Autodesk Inventor part; units mm, degrees
ref_plane "YZ Plane" through (0, 0, 0) normal (1, 0, 0) x (0, 1, 0)
ref_plane "XZ Plane" through (0, 0, 0) normal (0, 1, 0) x (-1, 0, 0)
ref_plane "XY Plane" through (0, 0, 0) normal (0, 0, 1) x (1, 0, 0)
sketch "Sketch1" plane through (0, 0, 0) normal (0, 0, 1) x (1, 0, 0)
  line L0 (2.54, -4.344) -> (-2.54, -4.344)
  line L1 (-2.54, -4.344) -> (-2.54, 4.344)
  line L2 (-2.54, 4.344) -> (2.54, 4.344)
  line L3 (2.54, 4.344) -> (2.54, -4.344)
  line L4 (2.54, -4.344) -> (-2.54, 4.344) construction
  line L5 (-2.54, -4.344) -> (2.54, 4.344) construction
  line L6 (4.445, 6.884) -> (-4.445, 6.884)
  line L7 (-4.445, 6.884) -> (-4.445, 1.804)
  line L8 (-4.445, 1.804) -> (4.445, 1.804)
  line L9 (4.445, 1.804) -> (4.445, 6.884)
  line L10 (4.445, 6.884) -> (-4.445, 1.804) construction
  line L11 (-4.445, 6.884) -> (4.445, 1.804) construction
  line L12 (3.8177, 1.5502) -> (-3.8177, 7.1379) construction
  line L13 (-4.445, -1.73) -> (4.445, 10.418) construction
  line L14 (6.985, 0) -> (-6.985, 0)
  line L15 (-6.985, 0) -> (-6.985, 25.4)
  line L16 (-6.985, 25.4) -> (6.985, 25.4)
  line L17 (6.985, 25.4) -> (6.985, 0)
  line L18 (6.985, 0) -> (-6.985, 25.4) construction
  line L19 (-6.985, 0) -> (6.985, 25.4) construction
  line L20 (0, 25.4) -> (0, 0) construction
  line L21 (-1.5875, 25.4) -> (1.5875, 25.4)
  line L22 (1.5875, 25.4) -> (1.5875, 13.234)
  line L23 (1.5875, 13.234) -> (-1.5875, 13.234)
  line L24 (-1.5875, 13.234) -> (-1.5875, 25.4)
  point P0 (0, 4.344)
  point P1 (0, 12.7)
  point P2 (2.54, 1.804)
  point P3 (2.54, 0)
  point P4 (-2.54, 0)
  point P5 (-2.54, 1.804)
  dimension "d0" = 5.08
  dimension "d1" = 8.89
  dimension "d2" = 5.08
  dimension "d3" = 8.89
  dimension "d4" = 8.89
  dimension "d5" = 13.97
  dimension "d6" = 25.4
  dimension "d7" = 0
  dimension "d8" = 3.175
  dimension "d9" = 1.5875
  dimension "d27" = 6.35
extrude "Extrusion1" add sketch "Sketch1" along normal blind 44.45 contours L3 L8 L9 L6 L7 L1 L14 L15 L16 L24 L23 L22 L17
sketch "Sketch2" plane through (0, 0, 0) normal (0, 0, -1) x (-1, 0, 0)
  line L0 (4.445, 6.884) -> (-4.445, 6.884)
  line L1 (4.445, 1.804) -> (4.445, 6.884)
  line L2 (2.54, 1.804) -> (4.445, 1.804)
  line L3 (2.54, 0) -> (2.54, 1.804)
  line L4 (6.985, 0) -> (2.54, 0)
  line L5 (6.985, 25.4) -> (6.985, 0)
  line L6 (1.5875, 25.4) -> (6.985, 25.4)
  line L7 (1.5875, 13.234) -> (1.5875, 25.4)
  line L8 (-1.5875, 13.234) -> (1.5875, 13.234)
  line L9 (-1.5875, 25.4) -> (-1.5875, 13.234)
  line L10 (-6.985, 25.4) -> (-1.5875, 25.4)
  line L11 (-6.985, 0) -> (-6.985, 25.4)
  line L12 (-2.54, 0) -> (-6.985, 0)
  line L13 (-2.54, 1.804) -> (-2.54, 0)
  line L14 (-4.445, 1.804) -> (-2.54, 1.804)
  line L15 (-4.445, 6.884) -> (-4.445, 1.804)
  line L16 (-1.5875, 25.4) -> (1.5875, 25.4)
  line L17 (1.5875, 25.4) -> (1.5875, 13.234)
  line L18 (1.5875, 13.234) -> (-1.5875, 13.234)
  line L19 (-1.5875, 13.234) -> (-1.5875, 25.4)
  point P0 (0, 0)
  point P1 (1.5875, 25.4)
extrude "Extrusion2" add sketch "Sketch2" against normal blind 6.35 contours L7 L8 L9 L16
sketch "Sketch3" plane through (6.985, 0, 0) normal (1, 0, 0) x (0, 0, -1)
  line L0 (0, 0) -> (0, 25.4)
  line L1 (0, 25.4) -> (-44.45, 25.4)
  line L2 (-44.45, 0) -> (-44.45, 25.4)
  line L3 (0, 0) -> (-44.45, 0)
  line L4 (-6.35, 25.4) -> (-6.35, 13.234)
  circle A0 centre (-3.175, 15.24) radius 3.175
  point P0 (0, 0)
  point P1 (0, 12.7)
  dimension "d14" = 6.35
  dimension "d15" = 3.175
  dimension "d16" = 10.16
extrude "Extrusion3" cut sketch "Sketch3" against normal through all contours A0
sketch "Sketch4" plane through (0, 0, 0) normal (0, 0, -1) x (-1, 0, 0)
  line L0 (4.445, 6.884) -> (-4.445, 6.884)
  line L1 (4.445, 1.804) -> (4.445, 6.884)
  line L2 (2.54, 1.804) -> (4.445, 1.804)
  line L3 (2.54, 0) -> (2.54, 1.804)
  line L4 (6.985, 0) -> (2.54, 0)
  line L5 (6.985, 25.4) -> (6.985, 15.24)
  line L6 (-6.985, 25.4) -> (6.985, 25.4)
  line L7 (-6.985, 0) -> (-6.985, 15.24)
  line L8 (-2.54, 0) -> (-6.985, 0)
  line L9 (-2.54, 1.804) -> (-2.54, 0)
  line L10 (-4.445, 1.804) -> (-2.54, 1.804)
  line L11 (-4.445, 6.884) -> (-4.445, 1.804)
  line L12 (-6.985, 0) -> (-6.985, 25.4)
  line L13 (-6.985, 12.7) -> (6.985, 12.7)
  line L14 (6.985, 25.4) -> (6.985, 0)
  line L15 (-6.985, 15.24) -> (6.985, 15.24)
  line L16 (-6.985, 15.24) -> (-6.985, 25.4)
  line L17 (6.985, 15.24) -> (6.985, 0)
  point P0 (0, 0)
  point P1 (-6.985, 12.7)
  point P2 (6.985, 12.7)
  dimension "d19" = 12.7
extrude "Extrusion4" add sketch "Sketch4" along normal blind 6.35
sketch "Sketch5" plane through (-6.985, 25.4, 44.45) normal (0, 1, 0) x (1, 0, 0)
  line L0 (0, 50.8) -> (0, 0)
  line L1 (13.97, 50.8) -> (13.97, 0)
  line L2 (0, 50.8) -> (13.97, 50.8)
  line L3 (13.97, 50.8) -> (13.97, 40.64)
  line L4 (13.97, 40.64) -> (0, 40.64)
  line L5 (0, 40.64) -> (0, 50.8)
  line L6 (0, 48.26) -> (13.97, 48.26)
  line L7 (13.97, 48.26) -> (13.97, 43.18)
  line L8 (13.97, 43.18) -> (0, 43.18)
  line L9 (0, 43.18) -> (0, 48.26)
  line L10 (0, 48.26) -> (13.97, 43.18) construction
  line L11 (13.97, 48.26) -> (0, 43.18) construction
  point P0 (6.985, 44.45)
  point P1 (6.985, 45.72)
  point P2 (0, 43.18)
  dimension "d22" = 10.16
  dimension "d23" = 5.08
  dimension "d24" = 5.08
  dimension "d29" = 0
extrude "Extrusion5" cut sketch "Sketch5" against normal blind 8.89 contours L6 L1 L8 L0
fillet "Fillet1" [suppressed]
properties part number "Drone_Launcher_Carriage"
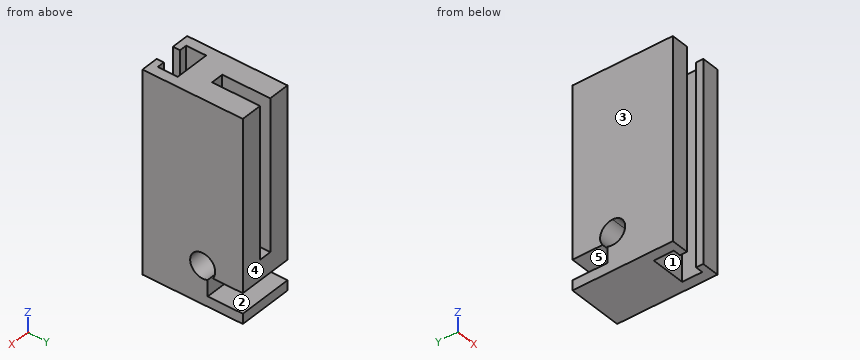
The listing builds one solid part. Answer for the finished solid, in the listing's coordinates (mm). Face numbers are marked on the shaded views. A direction names the side the tool comes from. Give positions to 0.01 mm unless a question says otherwise; leave off trailing zeros. Write each loop counter-clockwise with the first axis right and the second up, starting at its lowest first coordinate (ties: lowest second). Pieces come first, ordered by that corner, then holes. Notation, with made-up numbers: (73, 15.25) - (93, 15.25) arc R24 ccw to (93, 45.25) - close; hole circle Ø8 at (22.25, -37.75). An arc over 180 degrees is marked (long way). Use a Markdown table: item, result.
1. Find the intervals of material crossed by probe 1 along Z at (x, y) = (5, 20.75); probe 2 along Y at (x, z) = (-3.75, 39.5); probe 3 along X at (y, z) = (2.5, 31.5) (3 decimals), in increasing order. Write a range as from..to.
Values follow:
| item | result |
|---|---|
| probe 1 | z = -6.35..-3.81, 1.27..44.45 |
| probe 2 | y = 0..1.8, 6.88..25.4 |
| probe 3 | x = -6.985..-4.445, 4.445..6.985 |
2. Section D-D on z = 3.5 is taken. Write down the section's boundary in (x, y) (3 decimals), plus the area to 3 significant figures.
Values follow:
| item | result |
|---|---|
| outline | (-6.985, 0) - (-2.54, 0) - (-2.54, 1.804) - (-4.445, 1.804) - (-4.445, 6.884) - (4.445, 6.884) - (4.445, 1.804) - (2.54, 1.804) - (2.54, 0) - (6.985, 0) - (6.985, 12.082) - (-6.985, 12.082) - close; (-6.985, 18.398) - (6.985, 18.398) - (6.985, 25.4) - (-6.985, 25.4) - close |
| area | 212 mm² |
3. For a pull along X with two mould halves and no side action, classify the marked faces 1, 2 and 3 as released by +X, released by -X, zero draft, split by the parting line, or undercut.
Values follow:
| item | result |
|---|---|
| face 1 | undercut |
| face 2 | zero draft |
| face 3 | released by -X |
4. Section A-A on y = 2.75 is taken. Write down the section's boundary in (x, z) (3 decimals), plus the area to 3 significant figures.
Values follow:
| item | result |
|---|---|
| outline | (-6.985, -6.35) - (-4.445, -6.35) - (-4.445, 44.45) - (-6.985, 44.45) - close; (4.445, -6.35) - (6.985, -6.35) - (6.985, 44.45) - (4.445, 44.45) - close |
| area | 258 mm² |
5. A tool of negligible diameter and unlimited length cuts with its end or side. For the marked faces 4 and 5, from which of +Z, -Z, +X, -X, +Y, -Y can it reach the whole face along a straight path? Write none if from no direction.
Values follow:
| item | result |
|---|---|
| face 4 | +Z, -Z, +X, -X, +Y |
| face 5 | +X, -X, +Y |
6. Each of these flat-tipped pins is pushed along its axis until it touches: P1, Ø4, axis at x = -4.5, z = 19.5, coming from the -Y side; P2, Ø1, axis at x = -0.5, z = 0, coming from the +Y side; P3, Ø1.6, axis at x = 0, y = 20, coming from the +Z side. Where does it stop, or does it pass through?
Values follow:
| item | result |
|---|---|
| P1 | stops at y = 0 |
| P2 | stops at y = 16.51 |
| P3 | stops at z = 6.35 |
7. Section C-C on x = -5 is taken. Write down the section's boundary in (y, z) (3 decimals).
Values follow:
| item | result |
|---|---|
| outline | (0, -6.35) - (25.4, -6.35) - (25.4, -3.81) - (16.51, -3.81) - (16.51, 0.265) arc R3.175 cw (long way) to (17.78, 1.27) - (25.4, 1.27) - (25.4, 44.45) - (0, 44.45) - close |
